Model file for the job. Use its own axes, mm. A direction names the side the tool comes from. Coordinates: 2 decimals unless noted, no trailing zeros. Order: outer loops, then holes, each group sorted by start corner. A loop starts at its lowest first (then second) coordinate and runs counter-clockwise, first axis right, second up. Notation, with made-up numbers: (-24.75, 56.5) -> (17.25, 56.5) arc R23 cw to (17.25, 81.5) -> close; hole circle Ø1 at (40.25, -27.75). An arc over 180 degrees is marked (long way). Use CSV: the item, a comma, the result in double quotes. Start each with the question number.
(1) Tool access for faces 1 (the flat face through (-2.6, 1.5, 2.8)), 2 (the flat face through (0, 3, 3)), 3 (the flat face through (2.6, 1.5, 2.8)): list every direction of +Z, -Z, +X, -X, +Y, -Y with a clear straight run to the whole face (end or side of a thin tool).
(2) Cut at C-C on z = 0.55. Write the cut outline in (x, y), plus the area to 3 significant figures.
(3) Probe L1, parallel to Y at x = 0, z = 1.1; L2, parallel to Z at x = -3, y = -1.75; L3, parallel to X at y = 0.5, z = 2.95. List the from-to ranges inside material, lowest first.
(4) Pin check, flat tips, straight feed: pin 1 Ø3 at (y, z) = (2, 1.5) entering from +X; pin 2 Ø1 at (y, z) = (-2.5, 1) entering from -X; pin 3 Ø3 at (x, z) = (-0.5, 3) entering from -Y; pin 4 Ø1 at (x, y) = (-0.5, 1) entering from +Z. Stop position of each tip, or through.
(5) Pull direction Y, two halves, no side cores. Call faces 4 (the cylindrical face through (2.524, -1.485, 4.925)), 5 (the cylindrical face through (-2.524, 1.485, 4.925)), 6 (the cylindrical face through (-0.54, -2.44, 2.48)), 7 (the flat face through (2, 2, 0)): pulls with the +Y half, pulls with the -Y half, needs draft (parallel to the pull), parting line crosses it, or undercut.
(6) Cut at B-B on x = 0. Write the cut outline in (y, z).
(7) Cut at A-A on z = 3.7. Write the cut outline in (x, y).
Autodesk Inventor part; units mm, degrees
ref_plane "YZ Plane" through (0, 0, 0) normal (1, 0, 0) x (0, 1, 0)
ref_plane "XZ Plane" through (0, 0, 0) normal (0, 1, 0) x (-1, 0, 0)
ref_plane "XY Plane" through (0, 0, 0) normal (0, 0, 1) x (1, 0, 0)
sketch "草图1" plane through (0, 0, 0) normal (0, 0, 1) x (1, 0, 0)
  circle A0 centre (0, 0) radius 4
  dimension "d0" = 8
extrude "拉伸1" add sketch "草图1" along normal blind 1
sketch "草图2" plane through (0, 0, 1) normal (0, 0, 1) x (1, 0, 0)
  line L0 (1.7321, -3) -> (-1.7321, -3)
  line L1 (-1.7321, -3) -> (-3.4641, 0)
  line L2 (-3.4641, 0) -> (-1.7321, 3)
  line L3 (-1.7321, 3) -> (1.7321, 3)
  line L4 (1.7321, 3) -> (3.4641, 0)
  line L5 (3.4641, 0) -> (1.7321, -3)
  line L6 (0, 0) -> (0, 0.9644)
  point P0 (0, 3)
  dimension "d3" = 0.9644
  dimension "d4" = 6
extrude "拉伸2" add sketch "草图2" along normal blind 4
sketch "草图3" plane through (0, 0, 5) normal (0, 0, 1) x (1, 0, 0)
  circle A0 centre (0, 0) radius 2.5
  dimension "d7" = 5
extrude "拉伸3" cut sketch "草图3" against normal through all
thread "螺纹1"
fillet "圆角1" radius 0.25 7 edges at (-2.5981, 1.5, 5) (-2.5981, -1.5, 5) (0, 3, 5) (2.5981, 1.5, 5) (2.5981, -1.5, 5) (0, -3, 5) (-4, 0, 1)
chamfer "倒角1" distance 0.1 angle 45 1 edges at (-2.5, 0, 5)
properties part number "刀夹片紧固螺帽"
Outcome:
1,face 1,"+Z, -X, +Y"
1,face 2,"+Z, +X, -X, +Y"
1,face 3,"+Z, +X, +Y"
2,outline,"circle Ø8 at (0, 0); hole circle Ø5 at (0, 0)"
2,area,"30.6 mm2"
3,L1,"-3 to -2.5, 2.5 to 3"
3,L2,"0 to 1"
3,L3,"-3.18 to -2.45, 2.45 to 3.18"
4,pin 1,"x = 3.94"
4,pin 2,"x = -3.43"
4,pin 3,"y = -3"
4,pin 4,"through"
5,face 4,"pulls with the -Y half"
5,face 5,"pulls with the +Y half"
5,face 6,"undercut"
5,face 7,"needs draft"
6,outline,"(-4, 0) -> (-2.5, 0) -> (-2.5, 4.9) -> (-2.6, 5) -> (-2.75, 5) arc R0.25 ccw to (-3, 4.75) -> (-3, 1) -> (-3.75, 1) arc R0.25 ccw to (-4, 0.75) -> close; (2.5, 0) -> (4, 0) -> (4, 0.75) arc R0.25 ccw to (3.75, 1) -> (3, 1) -> (3, 4.75) arc R0.25 ccw to (2.75, 5) -> (2.6, 5) -> (2.5, 4.9) -> close"
7,outline,"(-3.46, 0) -> (-1.73, -3) -> (1.73, -3) -> (3.46, 0) -> (1.73, 3) -> (-1.73, 3) -> close; hole circle Ø5 at (0, 0)"
